Design review of the part shown in the three views and the two pictorial views. Dimensions are in mm from the part's minimum x, y and z. Give positions to 0.01 mm unless a question says otherwise; leave off trailing zeros. Loops run counter-clockwise (first coordinate to the right, second up) from the corner with the lowest first, then second, coordinate; pieces in that order, holes last. Notation, with made-up numbers: (-4, -15.75) - (40, -15.75) arc R19 cw to (40, -10.75) - close; hole circle Ø7 at (71, 60.5). An arc over 180 degrees is marked (long way). Answer as a JSON object with one key per item and string values.
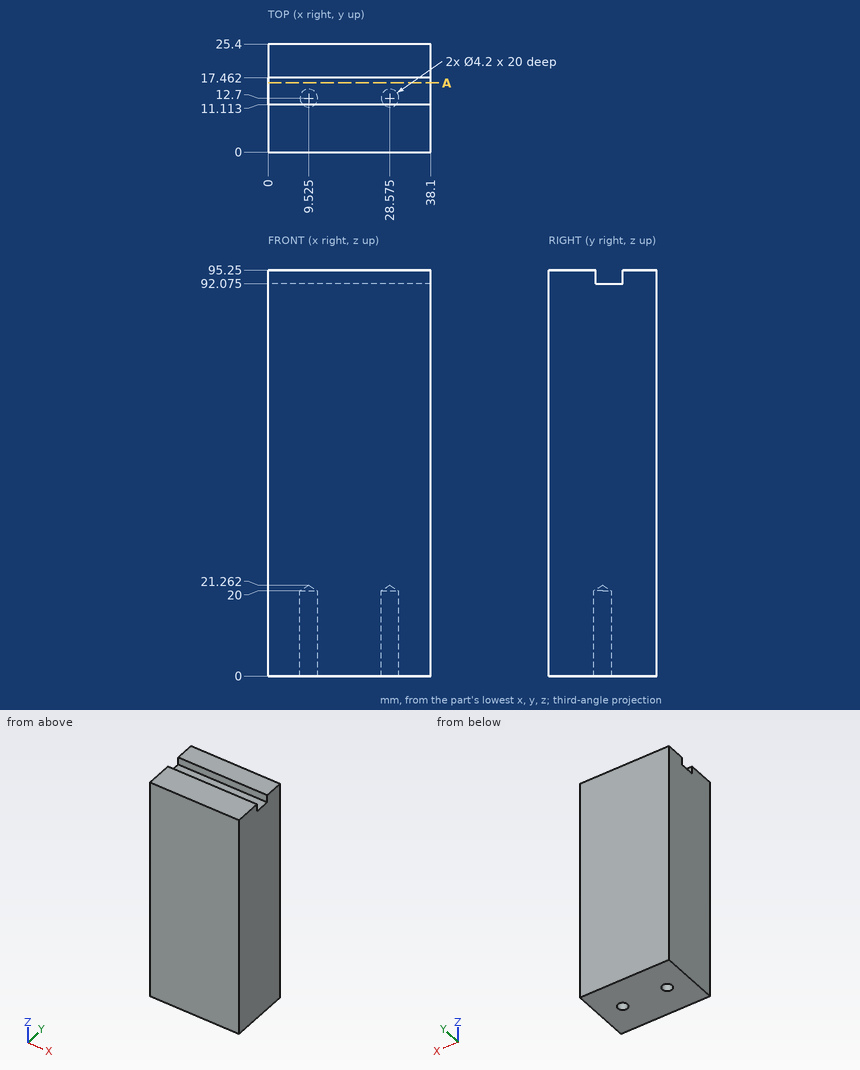
Q1. Consider section A-A, the plane y = 16.25. State the section outline as (x, z) points (1 decimal).
Results:
{"outline": "(0, 0) - (38.1, 0) - (38.1, 92.1) - (0, 92.1) - close"}
Q2. To check wall thickness, follow probe 1 along X at (y, z) = (12.7, 5.5) (1 decimal); probe 2 along Z at (x, y) = (31, 12.25) (1 decimal); probe 3 along Z at (x, y) = (29, 12) (1 decimal). State the ranges of each line that lie inside material, in increasing order. Write a range as [from, to].
Results:
{"probe 1": "x = [0, 7.4], [11.6, 26.5], [30.7, 38.1]", "probe 2": "z = [0, 92.1]", "probe 3": "z = [20.8, 92.1]"}
Q3. Clearance check with a flat-ended pin moving along its axis: pin 1 Ø3 at (x, y) = (19.5, 13.5) entering from +Z (1 decimal). State where the tip first meets the part, or that it passes through.
Results:
{"pin 1": "stops at z = 92.1"}
